For this review, take the finished solid that the model builds, in its own axes (mm). Round coordinates to 2 decimals unless told otherwise and drop trailing zeros. Loops run counter-clockwise (first coordinate to the right, second up) from the corner with the lowest first, then second, coordinate; pieces in that order, holes last.
1) Take a section at C-C (z = -127.5). State the section outline as (x, y) points, then the cut area to 3 significant figures.
2) Take a section at A-A (y = 182.5). State the section outline as (x, z) points, then the cut area to 3 significant figures.
3) Wall thickness on L1, parallel to Y at x = -1.1, z = -85.5; L2, parallel to Z at x = -2.3, y = 172.2; L3, parallel to Z at x = -3.9, y = 172.2: over which ranges is each line inside the solid? List them lowest first.
4) Insertion check: pin 1 (1.5 mm diameter, centred on x = -3.5, y = 235.5, fed in from +Z); pin 2 (3 mm diameter, centred on x = -4.5, y = 39, fed in from -Z). Each pin has a flat end and moves straight along its axis. Give the tip position at first contact, or say it passes through.
5) Take a section at B-B (x = -3.5). State the section outline as (y, z) points.
6) Take a section at D-D (y = 111). State the section outline as (x, z) points, then the cut area to 4 significant figures.
```python
from build123d import *

# Parameters (mm, degrees)
CROQUIS1_W              = 5
CROQUIS1_H              = 250
SALIENTE_EXTRUIR1_DEPTH = 330
CORTAR_EXTRUIR1_REACH   = 416.035
CORTAR_EXTRUIR2_REACH   = 416.035
CROQUIS3_W              = 200
CROQUIS3_H              = 80
CORTAR_EXTRUIR3_DEPTH   = 415.035022673
REDONDEO1_R             = 2.5
CROQUIS5_W              = 33.7
CROQUIS5_H              = 23.1
CORTAR_EXTRUIR4_DEPTH   = 415.035022673
CORTAR_EXTRUIR5_REACH   = 416.035
CROQUIS6_R              = 1


with BuildPart() as part:
    # Croquis1 → Saliente-Extruir1 (new body)
    with BuildSketch(Plane(origin=(0, 0, 0), x_dir=(1, 0, 0), z_dir=(0, 1, 0))):
        with Locations((-2.5, 125)):
            Rectangle(CROQUIS1_W, CROQUIS1_H)
    extrude(amount=SALIENTE_EXTRUIR1_DEPTH)

    # Croquis2 → Cortar-Extruir1 (cut, up to next)
    with BuildSketch(Plane(origin=(0, 330, 0), x_dir=(1, 0, 0), z_dir=(0, 1, 0)), mode=Mode.PRIVATE) as cortar_extruir1_sk1:
        Polygon((0, 250), (0, 245), (-5, 250), align=None)
    cortar_extruir1_tool1 = extrude(cortar_extruir1_sk1.sketch, amount=-CORTAR_EXTRUIR1_REACH, mode=Mode.PRIVATE) & part.part
    # Croquis2 → Cortar-Extruir1 (cut, up to next)
    with BuildSketch(Plane(origin=(0, 330, 0), x_dir=(1, 0, 0), z_dir=(0, 1, 0)), mode=Mode.PRIVATE) as cortar_extruir1_sk2:
        Polygon((-5, 0), (0, 5), (0, 0), align=None)
    cortar_extruir1_tool2 = extrude(cortar_extruir1_sk2.sketch, amount=-CORTAR_EXTRUIR1_REACH, mode=Mode.PRIVATE) & part.part
    add(cortar_extruir1_tool1.solids().sort_by_distance((-1.666667, 330, -248.333333))[0], mode=Mode.SUBTRACT)
    add(cortar_extruir1_tool2.solids().sort_by_distance((-1.666667, 330, -1.666667))[0], mode=Mode.SUBTRACT)

    # Croquis3 → Cortar-Extruir2 (cut, up to next)
    with BuildSketch(Plane.ZY.offset(5), mode=Mode.PRIVATE) as cortar_extruir2_sk1:
        with Locations((-125, 55)):
            Rectangle(CROQUIS3_W, CROQUIS3_H)
    cortar_extruir2_tool1 = extrude(cortar_extruir2_sk1.sketch, amount=-CORTAR_EXTRUIR2_REACH, mode=Mode.PRIVATE) & part.part
    add(cortar_extruir2_tool1.solids().sort_by_distance((-5, 55, -125))[0], mode=Mode.SUBTRACT)

    # Croquis4 → Cortar-Extruir3 (cut, through all)
    with BuildSketch(Plane.ZY.offset(5)):
        Polygon((-100, 198.5), (-100, 131.5), (-51, 131.5), (-36, 131.5), (-36, 161.5), (-51, 161.5), (-51, 198.5), align=None)
    extrude(amount=-CORTAR_EXTRUIR3_DEPTH, mode=Mode.SUBTRACT)

    # Redondeo1
    redondeo1_edges = [part.edges().sort_by_distance(p)[0] for p in [
        (-2.5, 131.5, -100),
        (-2.5, 198.5, -100),
        (-2.5, 198.5, -51),
        (-2.5, 161.5, -51),
        (-2.5, 161.5, -36),
        (-2.5, 131.5, -36),
    ]]
    fillet(redondeo1_edges, radius=REDONDEO1_R)

    # Croquis5 → Cortar-Extruir4 (cut, through all)
    with BuildSketch(Plane.ZY.offset(5)):
        with Locations((-75.5, 230.05)):
            Rectangle(CROQUIS5_W, CROQUIS5_H)
    extrude(amount=-CORTAR_EXTRUIR4_DEPTH, mode=Mode.SUBTRACT)

    # Croquis6 → Cortar-Extruir5 (cut, up to next)
    with BuildSketch(Plane.ZY.offset(5), mode=Mode.PRIVATE) as cortar_extruir5_sk1:
        with Locations((-230, 172.2)):
            Circle(CROQUIS6_R)
    cortar_extruir5_tool1 = extrude(cortar_extruir5_sk1.sketch, amount=-CORTAR_EXTRUIR5_REACH, mode=Mode.PRIVATE) & part.part
    # Croquis6 → Cortar-Extruir5 (cut, up to next)
    with BuildSketch(Plane.ZY.offset(5), mode=Mode.PRIVATE) as cortar_extruir5_sk2:
        with Locations((-160, 172.2)):
            Circle(CROQUIS6_R)
    cortar_extruir5_tool2 = extrude(cortar_extruir5_sk2.sketch, amount=-CORTAR_EXTRUIR5_REACH, mode=Mode.PRIVATE) & part.part
    add(cortar_extruir5_tool1.solids().sort_by_distance((-5, 172.2, -230))[0], mode=Mode.SUBTRACT)
    add(cortar_extruir5_tool2.solids().sort_by_distance((-5, 172.2, -160))[0], mode=Mode.SUBTRACT)


solid = part.part
```
Response:
1. outline: (-5, 0) - (0, 0) - (0, 15) - (-5, 15) - close; (-5, 95) - (0, 95) - (0, 330) - (-5, 330) - close
1. area: 1,250 mm2
2. outline: (-5, -250) - (0, -245) - (0, -100) - (-5, -100) - close; (-5, -51) - (0, -51) - (0, -5) - (-5, 0) - close
2. area: 980 mm2
3. L1: y = 0 to 15, 95 to 131.5, 198.5 to 218.5, 241.6 to 330
3. L2: z = -247.3 to -231, -229 to -161, -159 to -100, -51 to -2.7
3. L3: z = -248.9 to -231, -229 to -161, -159 to -100, -51 to -1.1
4. pin 1: stops at z = -0.75
4. pin 2: stops at z = -250
5. outline: (0, -248.5) - (330, -248.5) - (330, -1.5) - (0, -1.5) - close; hole (15, -225) - (95, -225) - (95, -25) - (15, -25) - close; hole (131.5, -97.5) arc R2.5 ccw to (134, -100) - (196, -100) arc R2.5 ccw to (198.5, -97.5) - (198.5, -53.5) arc R2.5 ccw to (196, -51) - (164, -51) arc R2.5 cw to (161.5, -48.5) - (161.5, -38.5) arc R2.5 ccw to (159, -36) - (134, -36) arc R2.5 ccw to (131.5, -38.5) - close; hole circle Ø2 at (172.2, -230); hole circle Ø2 at (172.2, -160); hole (218.5, -92.35) - (241.6, -92.35) - (241.6, -58.65) - (218.5, -58.65) - close
6. outline: (-5, -250) - (0, -245) - (0, -5) - (-5, 0) - close
6. area: 1,225 mm2
